from build123d import *

# Parameters (mm, degrees)
F0_R     = 1.75
F1_DEPTH = 1


with BuildPart() as f1:
    # F0 (on Top) → F1 (new body)
    with BuildSketch(Plane.XY):
        Polygon((12, 14), (-12, 14), (-25, 1), (-25, -1), (-12, -14), (12, -14), (25, -1), (25, 1), align=None)
        with Locations((-20, 0)):
            Circle(F0_R, mode=Mode.SUBTRACT)
        with BuildLine():
            Line((-16.25, 5.875), (-9.875, 12.25))
            Line((-9.875, 12.25), (10.125, 12.25))
            Line((10.125, 12.25), (16.25, 6.125))
            Line((16.25, 6.125), (16.25, -7.5))
            ThreePointArc((16.25, -7.5), (14.791493, -10.791493), (11.5, -12.25))
            Line((11.5, -12.25), (-11.5, -12.25))
            ThreePointArc((-11.5, -12.25), (-14.791493, -10.791493), (-16.25, -7.5))
            Line((-16.25, -7.5), (-16.25, 5.875))
        make_face(mode=Mode.SUBTRACT)
        with Locations((20, 0)):
            Circle(F0_R, mode=Mode.SUBTRACT)
    extrude(amount=F1_DEPTH)


solid = f1.part
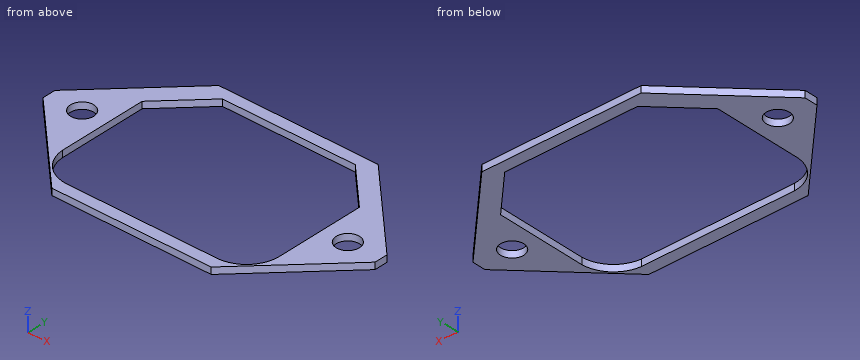
Part model, mm, in its own coordinate system. Coordinates: 2 decimals unless noted, no trailing zeros. Loops run counter-clockwise (first coordinate to the right, second up) from the corner with the lowest first, then second, coordinate; pieces in that order, holes last. Notation, with made-up numbers: M 72,41.5 L 108,41.5 A20 cw 108,55.5 Z; hole C -29,83 d10. An arc over 180 degrees is marked long. Use a Markdown table: item, result. Add a question column.
Q1. Cut at D-D (y = -10.75). Write the cut outline in (x, z), and give its area (3 significant figures).
Q2. Pin check, flat tip, straight feed: P1, Ø4.5, axis at x = 20, y = 0, coming from the +Z side. Stop position of the tip, or through.
Q3. Cut at B-B (x = 4). Write the cut outline in (y, z).
Q4. Cut at A-A (z = 0.8). Write the cut outline in (x, y) (3 decimals), and give its area (3 significant figures).
Q5. Cut at C-C (y = 0). Write the cut outline in (x, z), and give its area (3 significant figures).
Q6. Probe L1, parallel to Y at x = -6.5, z = 0.85; L2, parallel to Y at x = -20, z = 0.45; L3, parallel to X at y = 7, z = 0.9 (3 decimals). List the from-to ranges inside material, lowest first.
Worked out:
| question | item | result |
|---|---|---|
| 1 | outline | M -15.25,0 L -14.83,0 L -14.83,1 L -15.25,1 Z; M 14.83,0 L 15.25,0 L 15.25,1 L 14.83,1 Z |
| 1 | area | 0.835 mm2 |
| 2 | P1 | stops at z = 1 |
| 3 | outline | M -14,0 L -12.25,0 L -12.25,1 L -14,1 Z; M 12.25,0 L 14,0 L 14,1 L 12.25,1 Z |
| 4 | outline | M -25,-1 L -12,-14 L 12,-14 L 25,-1 L 25,1 L 12,14 L -12,14 L -25,1 Z; hole C -20,0 d3.5; hole M -16.25,-7.5 A5 ccw -11.5,-12.25 L 11.5,-12.25 A5 ccw 16.25,-7.5 L 16.25,6.125 L 10.125,12.25 L -9.875,12.25 L -16.25,5.875 Z; hole C 20,0 d3.5 |
| 4 | area | 296 mm2 |
| 5 | outline | M -25,0 L -21.75,0 L -21.75,1 L -25,1 Z; M -18.25,0 L -16.25,0 L -16.25,1 L -18.25,1 Z; M 16.25,0 L 18.25,0 L 18.25,1 L 16.25,1 Z; M 21.75,0 L 25,0 L 25,1 L 21.75,1 Z |
| 5 | area | 10.5 mm2 |
| 6 | L1 | y = -14 to -12.25, 12.25 to 14 |
| 6 | L2 | y = -6 to -1.75, 1.75 to 6 |
| 6 | L3 | x = -19 to -15.125, 15.375 to 19 |
